Geometry: final body of the model. Coordinates: model frame, mm. Round coordinates to 2 decimals unless told otherwise and drop trailing zeros. Loops run counter-clockwise (first coordinate to the right, second up) from the corner with the lowest first, then second, coordinate; pieces in that order, holes last. Notation, with made-up numbers: (34.25, 6) - (89.25, 6) arc R37 ccw to (89.25, 44) - close; hole circle Ø1 at (16, 32.5). An arc over 180 degrees is marked (long way). Return JSON: item names as keys, results as strings. Group by question number.
1. Section A-A on y = 39.5. Return loops of the section in (x, z).
2. Material intervals for probe 1 along X at (y, z) = (33, 0.7); probe 2 along Y at (x, z) = (57, 0.1); probe 3 along X at (y, z) = (91.5, 0.85), sorted ascending.
3. Draft query along X for faces 1 (the face through (47, 50, 0)), 2 (the face through (50.33, 99.5, 0.59)), 3 (the face through (31.443, 43.182, 0.592)). Return one class per face: +X half, -X half, draft (parallel to the pull), parting line (faces both ways), or undercut.
from build123d import *

# Parameters (mm, degrees)
SKETCH1_R           = 25
BOSS_EXTRUDE2_DEPTH = 1.2


with BuildPart() as part:
    # Sketch1 → Boss-Extrude2 (new body)
    # profile 1 of 2: a face of its own
    with BuildSketch(Plane.XY):
        with BuildLine():
            ThreePointArc((30.012612552, 44.909806232), (31.456939617, 43.153429969), (31.974033442, 40.939033386))
            Line((31.974033442, 40.939033386), (31.974033442, 24.710911787))
            Line((31.974033442, 24.710911787), (33.174033442, 24.710911787))
            Line((33.174033442, 24.710911787), (33.174033442, 25.910911787))
            Line((33.174033442, 25.910911787), (33.174033442, 40.939033386))
            ThreePointArc((33.174033442, 40.939033386), (32.532837099, 43.684885149), (30.741871538, 45.862791715))
            add(Edge.make_bspline(
                [(23.907304336, 52.680952793), (24.895982804, 51.393814611), (25.961184771, 50.183384061), (28.239708338, 47.910999007), (29.453038683, 46.849053267), (30.741871538, 45.862791715)],
                knots=[0, 0, 0, 0, 0.5, 0.5, 1, 1, 1, 1], degree=3))
            add(Edge.make_bspline(
                [(18.120262379, 63.710555688), (20.071106868, 57.700914274), (23.907304336, 52.680952793)],
                knots=[0, 0, 0, 1, 1, 1], degree=2))
            add(Edge.make_bspline(
                [(46.603584144, 110.619037792), (44.037564697, 110.136881177), (41.565586639, 109.399910271), (37.993900492, 107.925187439), (36.826238957, 107.371561991), (35.110219129, 106.445007697), (34.542851373, 106.119235257), (33.43252755, 105.44242724), (32.888321687, 105.090808098), (30.221191305, 103.267699747), (28.258194172, 101.603306881), (25.574408604, 98.792250251), (24.720125305, 97.796907394), (23.13911088, 95.742873652), (21.676894423, 93.618239495), (20.448442982, 91.354681184), (19.616276632, 89.604018307), (19.353780354, 89.011613552), (18.859214477, 87.808721777), (18.626764638, 87.196877672), (17.554889932, 84.128083475), (16.972551184, 81.619082003), (16.582490206, 78.416566694), (16.521549682, 77.772715441), (16.434385915, 76.478203987), (16.408151888, 75.825935146), (16.382947935, 73.870123777), (16.437042358, 72.576530522), (16.804915383, 68.725563933), (17.321982276, 66.197670032), (18.120262379, 63.710555688)],
                knots=[0, 0, 0, 0, 0.125, 0.125, 0.1875, 0.1875, 0.21875, 0.21875, 0.25, 0.25, 0.375, 0.375, 0.4375, 0.4375, 0.5, 0.5625, 0.5625, 0.59375, 0.59375, 0.625, 0.625, 0.75, 0.75, 0.78125, 0.78125, 0.8125, 0.8125, 0.875, 0.875, 1, 1, 1, 1], degree=3))
            Line((46.603584144, 110.619037792), (51.983858638, 111.235180692))
            add(Edge.make_bspline(
                [(90.774033442, 74.710911787), (90.774033442, 77.213730522), (90.515335522, 79.672340976), (89.755654029, 83.296748891), (89.439994282, 84.494215906), (88.870483209, 86.274007547), (88.663985761, 86.866022189), (88.223006775, 88.032185971), (87.988280683, 88.607381066), (86.7448936, 91.444712748), (85.529077181, 93.592089305), (83.374781409, 96.630024235), (82.596689336, 97.616371359), (80.959746623, 99.487050945), (80.098944413, 100.375243684), (78.294879964, 102.059787228), (77.351613047, 102.856132822), (75.874606211, 103.98147858), (75.371900236, 104.345043579), (74.345466112, 105.048759603), (73.820236229, 105.389804232), (71.161791528, 107.022391302), (68.937418065, 108.097420547), (65.460029321, 109.376653093), (64.277247909, 109.747085072), (62.466669313, 110.216566623), (61.856506608, 110.358699396), (60.636162144, 110.611249978), (60.024506885, 110.7220877), (56.958913569, 111.200109803), (54.483245165, 111.341092134), (51.983858638, 111.235180692)],
                knots=[0, 0, 0, 0, 0.125, 0.125, 0.1875, 0.1875, 0.21875, 0.21875, 0.25, 0.25, 0.375, 0.375, 0.4375, 0.4375, 0.5, 0.5, 0.5625, 0.5625, 0.59375, 0.59375, 0.625, 0.625, 0.75, 0.75, 0.8125, 0.8125, 0.84375, 0.84375, 0.875, 0.875, 1, 1, 1, 1], degree=3))
            Line((90.774033442, 74.710911787), (90.774033442, 25.910911787))
            Line((90.774033442, 25.910911787), (90.774033442, 24.710911787))
            Line((90.774033442, 24.710911787), (91.973979472, 24.710911787))
            Line((91.973979472, 24.710911787), (91.974010458, 74.710883533))
            add(Edge.make_bspline(
                [(91.974010458, 74.710883533), (91.974034887, 114.130812003), (51.933054654, 112.434101318)],
                knots=[0, 0, 0, 1.61385221, 1.61385221, 1.61385221], degree=2, weights=[1, 0.691721555, 1]))
            Line((51.933054654, 112.434101318), (46.381981502, 111.79839875))
            add(Edge.make_bspline(
                [(46.381981502, 111.79839875), (3.982488462, 103.83150821), (16.977674359, 63.34382334)],
                knots=[4.901152551, 4.901152551, 4.901152551, 6.588978479, 6.588978479, 6.588978479], degree=2, weights=[1, 0.664543961, 1]))
            ThreePointArc((16.977674359, 63.34382334), (17.041173685, 63.129657728), (17.095043921, 62.912869648))
            add(Edge.make_bspline(
                [(17.095043921, 62.912869648), (18.7559158, 56.98560233), (22.647992265, 52.31328285)],
                knots=[0.033678654, 0.033678654, 0.033678654, 0.963651852, 0.963651852, 0.963651852], degree=2))
            ThreePointArc((22.647992265, 52.31328285), (22.806145611, 52.135286834), (22.955645602, 51.949963291))
            add(Edge.make_bspline(
                [(22.955645602, 51.949963291), (26.0115243, 47.971583788), (30.012612552, 44.909806232)],
                knots=[0.647016148, 0.647016148, 0.647016148, 0.90960641, 0.90960641, 0.90960641], degree=2, weights=[1, 0.991393169, 1]))
        make_face()
    # profile 2 of 2: a face of its own
    with BuildSketch(Plane.XY):
        with BuildLine():
            Line((33.174033442, 25.910911787), (33.174033442, 24.710911787))
            Line((33.174033442, 24.710911787), (90.774033442, 24.710911787))
            Line((90.774033442, 24.710911787), (90.774033442, 25.910911787))
            Line((90.774033442, 25.910911787), (90.774033442, 74.710911787))
            add(Edge.make_bspline(
                [(90.774033442, 74.710911787), (90.774033442, 77.213730522), (90.515335522, 79.672340976), (89.755654029, 83.296748891), (89.439994282, 84.494215906), (88.870483209, 86.274007547), (88.663985761, 86.866022189), (88.223006775, 88.032185971), (87.988280683, 88.607381066), (86.7448936, 91.444712748), (85.529077181, 93.592089305), (83.374781409, 96.630024235), (82.596689336, 97.616371359), (80.959746623, 99.487050945), (80.098944413, 100.375243684), (78.294879964, 102.059787228), (77.351613047, 102.856132822), (75.874606211, 103.98147858), (75.371900236, 104.345043579), (74.345466112, 105.048759603), (73.820236229, 105.389804232), (71.161791528, 107.022391302), (68.937418065, 108.097420547), (65.460029321, 109.376653093), (64.277247909, 109.747085072), (62.466669313, 110.216566623), (61.856506608, 110.358699396), (60.636162144, 110.611249978), (60.024506885, 110.7220877), (56.958913569, 111.200109803), (54.483245165, 111.341092134), (51.983858638, 111.235180692)],
                knots=[0, 0, 0, 0, 0.125, 0.125, 0.1875, 0.1875, 0.21875, 0.21875, 0.25, 0.25, 0.375, 0.375, 0.4375, 0.4375, 0.5, 0.5, 0.5625, 0.5625, 0.59375, 0.59375, 0.625, 0.625, 0.75, 0.75, 0.8125, 0.8125, 0.84375, 0.84375, 0.875, 0.875, 1, 1, 1, 1], degree=3))
            Line((51.983858638, 111.235180692), (46.603584144, 110.619037792))
            add(Edge.make_bspline(
                [(46.603584144, 110.619037792), (44.037564697, 110.136881177), (41.565586639, 109.399910271), (37.993900492, 107.925187439), (36.826238957, 107.371561991), (35.110219129, 106.445007697), (34.542851373, 106.119235257), (33.43252755, 105.44242724), (32.888321687, 105.090808098), (30.221191305, 103.267699747), (28.258194172, 101.603306881), (25.574408604, 98.792250251), (24.720125305, 97.796907394), (23.13911088, 95.742873652), (21.676894423, 93.618239495), (20.448442982, 91.354681184), (19.616276632, 89.604018307), (19.353780354, 89.011613552), (18.859214477, 87.808721777), (18.626764638, 87.196877672), (17.554889932, 84.128083475), (16.972551184, 81.619082003), (16.582490206, 78.416566694), (16.521549682, 77.772715441), (16.434385915, 76.478203987), (16.408151888, 75.825935146), (16.382947935, 73.870123777), (16.437042358, 72.576530522), (16.804915383, 68.725563933), (17.321982276, 66.197670032), (18.120262379, 63.710555688)],
                knots=[0, 0, 0, 0, 0.125, 0.125, 0.1875, 0.1875, 0.21875, 0.21875, 0.25, 0.25, 0.375, 0.375, 0.4375, 0.4375, 0.5, 0.5625, 0.5625, 0.59375, 0.59375, 0.625, 0.625, 0.75, 0.75, 0.78125, 0.78125, 0.8125, 0.8125, 0.875, 0.875, 1, 1, 1, 1], degree=3))
            add(Edge.make_bspline(
                [(18.120262379, 63.710555688), (20.071106868, 57.700914274), (23.907304336, 52.680952793)],
                knots=[0, 0, 0, 1, 1, 1], degree=2))
            add(Edge.make_bspline(
                [(23.907304336, 52.680952793), (24.895982804, 51.393814611), (25.961184771, 50.183384061), (28.239708338, 47.910999007), (29.453038683, 46.849053267), (30.741871538, 45.862791715)],
                knots=[0, 0, 0, 0, 0.5, 0.5, 1, 1, 1, 1], degree=3))
            ThreePointArc((30.741871538, 45.862791715), (32.532837099, 43.684885149), (33.174033442, 40.939033386))
            Line((33.174033442, 40.939033386), (33.174033442, 25.910911787))
        make_face()
        with Locations((53.585400153, 74.710911787)):
            Circle(SKETCH1_R, mode=Mode.SUBTRACT)
    extrude(amount=BOSS_EXTRUDE2_DEPTH)


solid = part.part
Taken from the geometry:
{
 "1": {"outline": "(31.97, 0) - (91.97, 0) - (91.97, 1.2) - (31.97, 1.2) - close"},
 "2": {"probe 1": "31.97 to 91.97", "probe 2": "24.71 to 49.95, 99.48 to 112.32", "probe 3": "19.2 to 35.06, 72.11 to 87.97"},
 "3": {"face 1": "draft", "face 2": "undercut", "face 3": "-X half"}
}
